from build123d import *

# Parameters (mm, degrees)
F0_R     = 3.175
F0_W     = 5.842
F0_H     = 12.7
F1_DEPTH = 3.175
F4_DEPTH = 2.54


with BuildPart() as f1:
    # F0 (on Front) → F1 (new body, symmetric)
    with BuildSketch(Plane.XZ):
        with BuildLine():
            Line((-0.9398, 0), (0, 0))
            Line((0, 0), (0, 12.7))
            Line((0, 12.7), (5.842, 12.7))
            Line((5.842, 12.7), (5.842, 15.24))
            Line((5.842, 15.24), (-0.508, 15.24))
            Line((-0.508, 15.24), (-10.88063, 3.847543))
            ThreePointArc((-10.88063, 3.847543), (-4.591961, 5.329721), (-0.9398, 0))
        make_face()
        with BuildLine():
            ThreePointArc((-8.182663, -5.506983), (-3.195791, -4.549339), (-0.9398, 0))
            ThreePointArc((-0.9398, 0), (-4.591961, 5.329721), (-10.88063, 3.847543))
            ThreePointArc((-10.88063, 3.847543), (-12.145978, -1.583727), (-8.182663, -5.506983))
        make_face()
        with Locations((-6.6548, 0)):
            Circle(F0_R, mode=Mode.SUBTRACT)
        with BuildLine():
            Line((0, -7.777189), (0, 0))
            Line((0, 0), (-0.9398, 0))
            ThreePointArc((-0.9398, 0), (-3.195791, -4.549339), (-8.182663, -5.506983))
            Line((-8.182663, -5.506983), (0, -7.777189))
        make_face()
        Polygon((5.842, 0), (0, 0), (0, -7.777189), (5.842, -9.398), align=None)
        with Locations((2.921, 6.35)):
            Rectangle(F0_W, F0_H)
    extrude(amount=F1_DEPTH, both=True)

    # F0 (on Front) → F2 (revolve)
    with BuildSketch(Plane.XZ):
        Polygon((5.842, 12.7), (5.842, 0), (66.294, 0), (66.294, 12.7), (56.134, 12.7), (56.134, 10.16), (10.16, 10.16), (10.16, 12.7), align=None)
        with Locations((2.921, 6.35)):
            Rectangle(F0_W, F0_H)
    revolve(axis=Axis((33.147, 0, 0), (-1, 0, 0)))

    # F3 (on face) → F4 (join)
    with BuildSketch(Plane.YZ.offset(66.294)):
        Polygon((0.490244, 2.458155), (-4.588165, 1.773549), (-4.588165, -7.711818), (0.490244, -7.711818), align=None)
    extrude(amount=F4_DEPTH)


solid = f1.part
Read the model definition and answer for the solid it produces. Units are mm, in the model's axes. A direction names the side the tool comes from. Give positions to 0.01 mm unless a question says otherwise; leave off trailing zeros. Write each loop counter-clockwise with the first axis right and the second up, starting at its lowest first coordinate (ties: lowest second). Pieces come first, ordered by that corner, then holes. Notation, with made-up numbers: (74, -18) - (116, -18) arc R19 ccw to (116, -13) - close; hole circle Ø4 at (6.5, 83.5). An arc over 180 degrees is marked (long way). Return JSON: item names as keys, results as strings.
Q1. A cutting plane is placed at B-B, the plane y = -8. Determine the outline of the cut face in (x, z).
Reply:
{"outline": "(0, -9.86) - (10.16, -9.86) - (10.16, -6.26) - (56.13, -6.26) - (56.13, -9.86) - (66.29, -9.86) - (66.29, 9.86) - (56.13, 9.86) - (56.13, 6.26) - (10.16, 6.26) - (10.16, 9.86) - (0, 9.86) - close"}
Q2. Given P1, Ø5, axis at x = 11, y = -9, coming from the -Z side; P2, Ø1.5, axis at x = -1.5, z = 9.5, coming from the -Y side (3 decimals); P3, Ø1.5, axis at y = -0.5, z = 13.5, coming from the +X side; P4, Ø10, axis at x = 59.5, y = -2, coming from the -Z side, each flat-ended and moving along its own axis, determine where each tip first touches the part or whether it passes through.
Reply:
{"P1": "z = -10.82", "P2": "y = -3.175", "P3": "x = 5.84", "P4": "z = -12.7"}
Q3. A cutting plane is placed at A-A, the plane z = 0. Determine the outline of the cut face in (x, y) (3 decimals), and give its area (3 significant figures).
Reply:
{"outline": "(-12.37, -3.175) - (-9.83, -3.175) - (-9.83, 3.175) - (-12.37, 3.175) - close; (-3.48, -3.175) - (0, -3.175) - (0, -12.7) - (10.16, -12.7) - (10.16, -10.16) - (56.134, -10.16) - (56.134, -12.7) - (66.294, -12.7) - (66.294, -4.588) - (68.834, -4.588) - (68.834, 0.49) - (66.294, 0.49) - (66.294, 12.7) - (56.134, 12.7) - (56.134, 10.16) - (10.16, 10.16) - (10.16, 12.7) - (0, 12.7) - (0, 3.175) - (-3.48, 3.175) - close", "area": "1,500 mm²"}
Q4. Consider line 1 along X through (y, z) = (3.5, -2.25); line 2 along Y through (x, z) = (-7.5, 3.5) (3 decimals); line 3 along X through (y, z) = (2.5, -4.5). Determine where each line is inside the solid, lowest interval first. Write a range as [from, to].
Reply:
{"line 1": "[0, 66.29]", "line 2": "[-3.175, 3.175]", "line 3": "[-10.18, 66.29]"}
Q5. For faces 1 (the face through (0, -5, 0)), 2 (the face through (56.134, 9, -6)), 3 (the face through (68, -2, -7.712)), determine the directions among +Z, -Z, +X, -X, +Y, -Y from which every point of the face is accessible in a straight line to the end or side of a thin tool.
Reply:
{"face 1": "-Z, -X", "face 2": "none", "face 3": "-Z, +X, +Y, -Y"}
Q6. A cutting plane is placed at C-C, the plane x = 57.5. Determine the outline of the cut face in (y, z), and give its area (3 significant figures).
Reply:
{"outline": "circle Ø25.4 at (0, 0)", "area": "507 mm²"}
Q7. A cutting plane is placed at D-D, the plane x = 14. Determine the outline of the cut face in (y, z), and give its area (3 significant figures).
Reply:
{"outline": "circle Ø20.32 at (0, 0)", "area": "324 mm²"}
Q8. For a pull along X with two mould halves and no side action, classify faces 4 (the face through (32.825, 10.074, -1.323)), 5 (the face through (68, -4.588, -3)), 6 (the face through (68.834, -2, -3)) as released by +X, released by -X, zero draft, split by the parting line, or undercut.
Reply:
{"face 4": "undercut", "face 5": "zero draft", "face 6": "released by +X"}
